Drawing for the job (mm, zero at the part's lowest x, y, z). A direction names the side the tool comes from. Round coordinates to 2 decimals unless told otherwise and drop trailing zeros. Write each loop counter-clockwise with the first axis right and the second up, starting at its lowest first coordinate (ties: lowest second). Pieces come first, ordered by that corner, then holes. Notation, with made-up numbers: (52.5, 76) - (56.5, 76) arc R32 ccw to (56.5, 108) - close; hole circle Ø7 at (47.25, 43.25). An arc over 180 degrees is marked (long way). Answer in a Markdown table with one row per item.
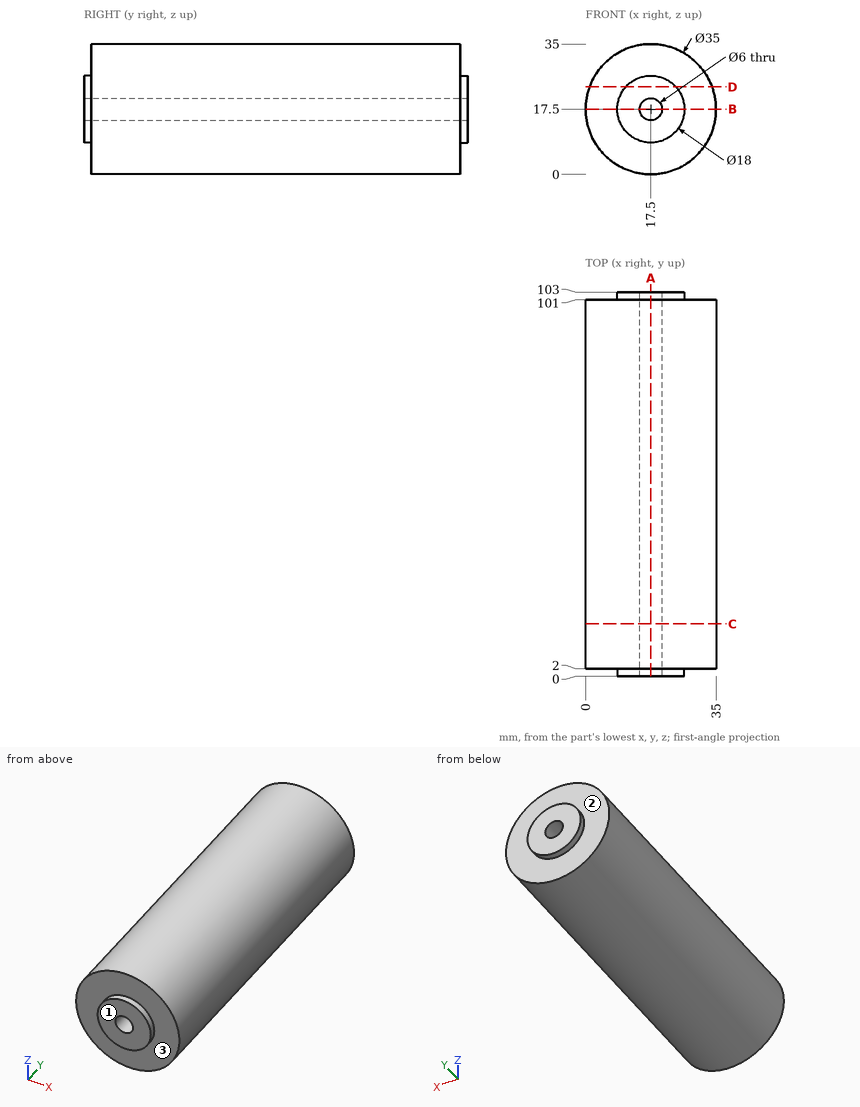
Q1. Saw through at D-D on z = 23.5. List the corners of the cut face in (x, y).
Computed:
| item | result |
|---|---|
| outline | (1.06, 2) - (10.79, 2) - (10.79, 0) - (24.21, 0) - (24.21, 2) - (33.94, 2) - (33.94, 101) - (24.21, 101) - (24.21, 103) - (10.79, 103) - (10.79, 101) - (1.06, 101) - close |
Q2. Saw through at A-A on x = 17.5. List the corners of the cut face in (y, z), then the cut area to 3 significant figures.
Computed:
| item | result |
|---|---|
| outline | (0, 8.5) - (2, 8.5) - (2, 0) - (101, 0) - (101, 8.5) - (103, 8.5) - (103, 14.5) - (0, 14.5) - close; (0, 20.5) - (103, 20.5) - (103, 26.5) - (101, 26.5) - (101, 35) - (2, 35) - (2, 26.5) - (0, 26.5) - close |
| area | 2,920 mm2 |
Q3. Drill centre lines: line 1 (X direction, y = 61.5, z = 17.5); line 2 (Y direction, x = 29, z = 11). Where is each one in solid material? Low to high.
Computed:
| item | result |
|---|---|
| line 1 | x = 0 to 14.5, 20.5 to 35 |
| line 2 | y = 2 to 101 |
Q4. Saw through at C-C on y = 14. List the corners of the cut face in (x, z).
Computed:
| item | result |
|---|---|
| outline | circle Ø35 at (17.5, 17.5); hole circle Ø6 at (17.5, 17.5) |
Q5. Flat gauge pins, fed straight in: pin 1 (3 mm diameter, centred on x = 12, y = 17.5, fed in from -Z); pin 2 (5.5 mm diameter, centred on x = 17.5, z = 17.5, fed in from +Y); pin 3 (5 mm diameter, centred on x = 30, z = 28, fed in from -Y); pin 4 (12 mm diameter, centred on x = 30.5, y = 14.5, fed in from +Z). Where does each tip first touch, or does it go through?
Computed:
| item | result |
|---|---|
| pin 1 | stops at z = 0.46 |
| pin 2 | passes through |
| pin 3 | stops at y = 2 |
| pin 4 | stops at z = 33.54 |
Q6. 3-axis set-ups, long thin cutter, end or side, ignore diameter. For the marked faces 1, 2 and 3: which of +Z, -Z, +X, -X, +Y, -Y reach the whole face in a straight line?
Computed:
| item | result |
|---|---|
| face 1 | +Z, -Z, +X, -X, -Y |
| face 2 | +Y |
| face 3 | -Y |
Q7. Saw through at B-B on z = 17.5. List the corners of the cut face in (x, y), then the cut area to 3 significant figures.
Computed:
| item | result |
|---|---|
| outline | (0, 2) - (8.5, 2) - (8.5, 0) - (14.5, 0) - (14.5, 103) - (8.5, 103) - (8.5, 101) - (0, 101) - close; (20.5, 0) - (26.5, 0) - (26.5, 2) - (35, 2) - (35, 101) - (26.5, 101) - (26.5, 103) - (20.5, 103) - close |
| area | 2,920 mm2 |
